Can you work these out from the drawing? Everything is in mm from the part's minimum corner. A direction names the side the tool comes from. Round coordinates to 2 decimals unless told otherwise and drop trailing zeros. Write each loop counter-clockwise with the first axis right and the second up, starting at its lowest first coordinate (ties: lowest second). Pieces come first, ordered by that corner, then holes. Notation, with made-up numbers: (39.25, 28) -> (96.25, 28) arc R14 cw to (96.25, 50) -> close; hole circle Ø3 at (29, -30.75). An arc over 180 degrees is marked (long way). One line per question, with ' | ' between items. Start each with the question number.
1. For the marked faces 4, 5, 6, 7 and 8, which set-ups out of +Z, -Z, +X, -X, +Y, -Y let a thin tool reach every point of the face, with its end or its side?
2. For pin 1 Ø2 at (y, z) = (9.5, 5.5) entering from -X; pin 2 Ø1.5 at (x, z) = (27.5, 3.5) entering from -Y; pin 3 Ø4 at (x, z) = (5.46, 5.3) entering from +Y, each with a flat end and sliding along its axis, tell me the tip position at first contact or that it passes through.
3. Thinking about a two-plate mould opening in Z: for the marked faces 1, 2 and 3, which applies, released by +Z, released by -Z, zero draft, split by the parting line, or undercut?
4. If I drill on line 1 along X through (y, z) = (9.25, 5.5); line 2 along X through (y, z) = (2, 1.25); line 3 along Y through (x, z) = (38.5, 0.5), over which ranges is the centre line in solid material (lowest first)? Write a range as [from, to].
5. Imagine slicing it at C-C, the plane x = 43.5. List the corners of the cut face in (y, z) for me (1 decimal).
6. Imagine slicing it at B-B, the plane z = 2.75. List the corners of the cut face in (x, y) for me, and give its area (3 significant figures).
7. Imagine slicing it at A-A, the plane y = 7.75. List the corners of the cut face in (x, z) for me, and give its area (3 significant figures).
8. Imagine slicing it at D-D, the plane z = 6. List the corners of the cut face in (x, y) for me, and give its area (3 significant figures).
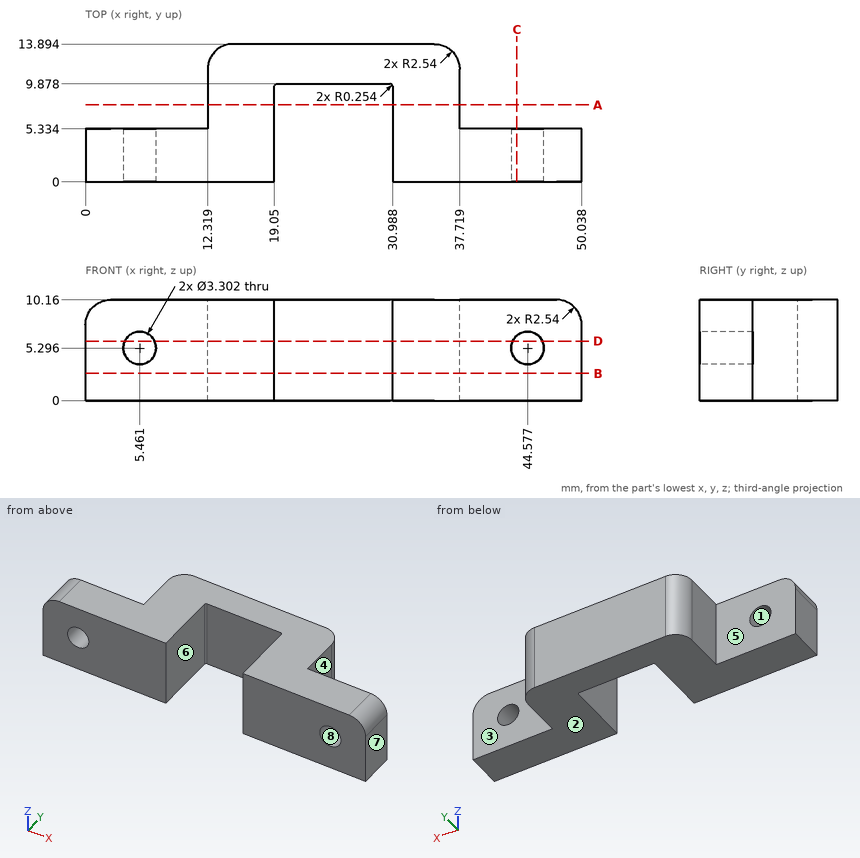
Geometry results:
1) face 4: +Z, -Z, +X, +Y | face 5: +Z, -Z, -X, +Y | face 6: +Z, -Z, -Y | face 7: +Z, -Z, +X, +Y, -Y | face 8: +Y, -Y
2) pin 1: stops at x = 12.32 | pin 2: stops at y = 9.88 | pin 3: stops at y = 5.33
3) face 1: undercut | face 2: released by -Z | face 3: zero draft
4) line 1: x = [12.32, 19.05], [30.99, 37.72] | line 2: x = [0, 19.05], [30.99, 50.04] | line 3: y = [0, 5.33]
5) outline: (0, 0) -> (5.3, 0) -> (5.3, 4) -> (0, 4) -> close; (0, 6.5) -> (5.3, 6.5) -> (5.3, 10.2) -> (0, 10.2) -> close
6) outline: (0, 0) -> (19.05, 0) -> (19.05, 9.62) arc R0.25 cw to (19.3, 9.88) -> (30.73, 9.88) arc R0.25 cw to (30.99, 9.62) -> (30.99, 0) -> (50.04, 0) -> (50.04, 5.33) -> (37.72, 5.33) -> (37.72, 11.35) arc R2.54 ccw to (35.18, 13.89) -> (14.86, 13.89) arc R2.54 ccw to (12.32, 11.35) -> (12.32, 5.33) -> (0, 5.33) -> close | area: 364 mm2
7) outline: (12.32, 0) -> (19.05, 0) -> (19.05, 10.16) -> (12.32, 10.16) -> close; (30.99, 0) -> (37.72, 0) -> (37.72, 10.16) -> (30.99, 10.16) -> close | area: 137 mm2
8) outline: (0, 0) -> (3.97, 0) -> (3.97, 5.33) -> (0, 5.33) -> close; (6.95, 0) -> (19.05, 0) -> (19.05, 9.62) arc R0.25 cw to (19.3, 9.88) -> (30.73, 9.88) arc R0.25 cw to (30.99, 9.62) -> (30.99, 0) -> (43.08, 0) -> (43.08, 5.33) -> (37.72, 5.33) -> (37.72, 11.35) arc R2.54 ccw to (35.18, 13.89) -> (14.86, 13.89) arc R2.54 ccw to (12.32, 11.35) -> (12.32, 5.33) -> (6.95, 5.33) -> close; (46.07, 0) -> (50.04, 0) -> (50.04, 5.33) -> (46.07, 5.33) -> close | area: 332 mm2
